The listing builds one solid part. Answer for the finished solid, in the listing's coordinates (mm). Round coordinates to 2 decimals unless told otherwise and drop trailing zeros. Loops run counter-clockwise (first coordinate to the right, second up) from the corner with the lowest first, then second, coordinate; pieces in that order, holes last. Notation, with made-up numbers: (13.5, 16) -> (68.5, 16) arc R25 cw to (68.5, 38) -> close; hole circle Ø6 at (26, 15.5). An arc over 180 degrees is marked (long way). One line per question, with ' | ' between items.
from build123d import *

# Parameters (mm, degrees)
F0_W     = 177.8
F0_H     = 127
F1_DEPTH = 25.4
F2_R     = 38.1
F3_DEPTH = 50.801
F4_R     = 8.929269
F5_DEPTH = 50.801


with BuildPart() as f1:
    # F0 (on Front) → F1 (new body, symmetric)
    with BuildSketch(Plane.XZ):
        Rectangle(F0_W, F0_H)
    extrude(amount=F1_DEPTH, both=True)

    # F2 (on face) → F3 (cut, through all)
    with BuildSketch(Plane(origin=(0, 25.4, 0), x_dir=(-1, 0, 0), z_dir=(0, 1, 0))):
        Circle(F2_R)
    extrude(amount=-F3_DEPTH, mode=Mode.SUBTRACT)

    # F4 (on face) → F5 (cut, through all)
    with BuildSketch(Plane.XZ.offset(25.4)):
        with Locations((-70.516594, 43.921053)):
            Circle(F4_R)
    extrude(amount=-F5_DEPTH, mode=Mode.SUBTRACT)


solid = f1.part
Q1. Find the intervals of material crossed by line 1 (Z direction, x = 0, y = 9.5); line 2 (X direction, y = 10, z = 0.5); line 3 (Z direction, x = -35, y = -19.5), in increasing order. Write a range as from..to.
Numbers:
line 1: -63.5..-38.1, 38.1..63.5 | line 2: -88.9..-38.1, 38.1..88.9 | line 3: -63.5..-15.05, 15.05..63.5
Q2. A cutting plane is placed at B-B on x = 0. Give the vertices of the cut face in (y, z), plus the area to 3 significant figures.
Numbers:
outline: (-25.4, -63.5) -> (25.4, -63.5) -> (25.4, -38.1) -> (-25.4, -38.1) -> close; (-25.4, 38.1) -> (25.4, 38.1) -> (25.4, 63.5) -> (-25.4, 63.5) -> close | area: 2,580 mm^2
Q3. For a pull along X with two mould halves and no side action, classify faces 1 (the face through (-88.9, 0, -1)), 2 (the face through (-71.679, -0.356, 52.774)), 3 (the face through (38.3, -25.4, 0.9)), 4 (the face through (30.235, 0.356, -23.183)) as pulls with the +X half, pulls with the -X half, needs draft (parallel to the pull), parting line crosses it, or undercut.
Numbers:
face 1: pulls with the -X half | face 2: undercut | face 3: needs draft | face 4: undercut
Q4. A cutting plane is placed at C-C on y = -17.5. Give the vertices of the cut face in (x, z).
Numbers:
outline: (-88.9, -63.5) -> (88.9, -63.5) -> (88.9, 63.5) -> (-88.9, 63.5) -> close; hole circle Ø17.86 at (-70.52, 43.92); hole circle Ø76.2 at (0, 0)
Q5. A cutting plane is placed at A-A on z = 0. Give the vertices of the cut face in (x, y), plus the area to 3 significant figures.
Numbers:
outline: (-88.9, -25.4) -> (-38.1, -25.4) -> (-38.1, 25.4) -> (-88.9, 25.4) -> close; (38.1, -25.4) -> (88.9, -25.4) -> (88.9, 25.4) -> (38.1, 25.4) -> close | area: 5,160 mm^2
